Can you work these out from the model? Positions are in its coordinate system, mm. Face numbers are marked on the shaded views. A direction names the side the tool comes from. Round coordinates to 2 decimals unless told otherwise and drop trailing zeros. Loops run counter-clockwise (first coordinate to the right, second up) from the corner with the lowest first, then second, coordinate; pieces in that order, holes last.
```python
from build123d import *

# Parameters (mm, degrees)
F0_W      = 20
F0_H      = 20
F1_DEPTH  = 70
F0_W_2    = 5
F0_R      = 2.5
F2_DEPTH  = 5
F3_W      = 18
F3_H      = 18
F4_DEPTH  = 20
F5_W      = 20
F5_H      = 20
F6_DEPTH  = 2
F7_SIZE   = 2
F8_SIZE   = 1
F9_W      = 18
F9_H      = 18
F10_DEPTH = 20
F11_SIZE  = 1


with BuildPart() as f1:
    # F0 (on Top) → F1 (new body)
    with BuildSketch(Plane.XY):
        with Locations((15, 10)):
            Rectangle(F0_W, F0_H)
    extrude(amount=F1_DEPTH)

    # F0 (on Top) → F2 (join)
    with BuildSketch(Plane.XY):
        with Locations((2.5, 10)):
            Rectangle(F0_W_2, F0_H)
        with BuildLine():
            ThreePointArc((0, 20), (-10, 10), (0, 0))
            Line((0, 0), (0, 20))
        make_face()
        with Locations((-4, 10)):
            Circle(F0_R, mode=Mode.SUBTRACT)
        with Locations((15, 10)):
            Rectangle(F0_W, F0_H)
        with Locations((27.5, 10)):
            Rectangle(F0_W_2, F0_H)
        with BuildLine():
            Line((30, 20), (30, 0))
            ThreePointArc((30, 0), (40, 10), (30, 20))
        make_face()
        with Locations((34, 10)):
            Circle(F0_R, mode=Mode.SUBTRACT)
    extrude(amount=-F2_DEPTH)

    # F3 (on face) → F4 (join)
    with BuildSketch(Plane.XY.offset(70)):
        with Locations((15, 10)):
            Rectangle(F3_W, F3_H)
    extrude(amount=F4_DEPTH)

    # F5 (on face) → F6 (join)
    with BuildSketch(Plane.XZ):
        with Locations((15, 58)):
            Rectangle(F5_W, F5_H)
    extrude(amount=F6_DEPTH)

    # F7
    f7_edges = [f1.edges().sort_by_distance(p)[0] for p in [
        (31.5, 10, 0),
        (-6.5, 10, 0),
    ]]
    chamfer(f7_edges, length=F7_SIZE)

    # F8
    f8_edges = [f1.edges().sort_by_distance(p)[0] for p in [
        (24, 19, 80),
        (6, 19, 80),
        (15, 19, 90),
        (6, 10, 90),
        (24, 10, 90),
        (15, 1, 90),
        (24, 1, 80),
        (6, 1, 80),
    ]]
    chamfer(f8_edges, length=F8_SIZE)

    # F9 (on face) → F10 (join)
    with BuildSketch(Plane.XZ.offset(2)):
        with Locations((15, 58)):
            Rectangle(F9_W, F9_H)
    extrude(amount=F10_DEPTH)

    # F11
    f11_edges = [f1.edges().sort_by_distance(p)[0] for p in [
        (24, -12, 67),
        (15, -22, 67),
        (6, -12, 67),
        (24, -22, 58),
        (24, -12, 49),
        (6, -12, 49),
        (6, -22, 58),
        (15, -22, 49),
    ]]
    chamfer(f11_edges, length=F11_SIZE)


solid = f1.part
```
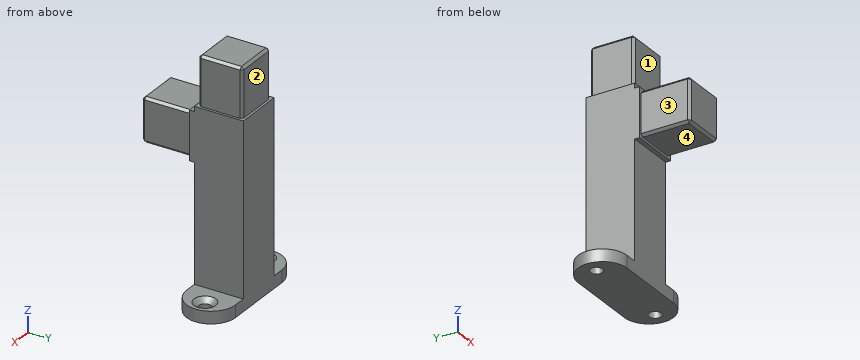
(1) Which directions (+Z, -Z, +X, -X, +Y, -Y) give clear straight access to the entire face, cutting with the end or side of a thin tool? Please do the marked faces 1, 2, 3 and 4.
(2) Suppose I cut it at C-C (y = -6). Write out the boundary of the cut face in (x, z).
(3) For pin 1 (4 mm diameter, centred on y = 9.5, z = 11, fed in from +X); pin 2 (5 mm diameter, centred on y = 10, z = 82.5, fed in from -X); pin 3 (24 mm diameter, centred on y = 5, z = 30.5, fed in from -X), each with a flat end and sliding along its axis, tell me the tip position at first contact or that it passes through.
(4) Suppose I cut it at D-D (x = 14). Write out the boundary of the cut face in (y, z), then the cut area to 3 significant figures.
(5) Suppose I cut it at B-B (x = -4). Write out the boundary of the cut face in (y, z).
(6) Suppose I cut it at A-A (y = 10). Write out the boundary of the cut face in (x, z).
(7) If I drill on line 1 (Z direction, x = 30.5, y = 7); line 2 (Y direction, x = 23, z = 5.5); line 3 (Y direction, x = 18.5, z = 81.5), over which ranges is the centre line in solid material (lowest first)?
Check result:
1. face 1: +Z, +X, -X, -Y
1. face 2: +Z, +X, -X, +Y
1. face 3: +Z, -Z, -X, -Y
1. face 4: -Z, +X, -X, -Y
2. outline: (6, 50) - (7, 49) - (23, 49) - (24, 50) - (24, 66) - (23, 67) - (7, 67) - (6, 66) - close
3. pin 1: stops at x = 25
3. pin 2: stops at x = 6
3. pin 3: stops at x = 5
4. outline: (-22, 50) - (-21, 49) - (-2, 49) - (-2, 48) - (0, 48) - (0, -5) - (20, -5) - (20, 70) - (19, 70) - (19, 89) - (18, 90) - (2, 90) - (1, 89) - (1, 70) - (0, 70) - (0, 68) - (-2, 68) - (-2, 67) - (-21, 67) - (-22, 66) - close
4. area: 2,260 mm2
5. outline: (0.83, -5) - (7.5, -5) - (7.5, -2) - (5.5, 0) - (0.83, 0) - close; (12.5, -5) - (19.17, -5) - (19.17, 0) - (14.5, 0) - (12.5, -2) - close
6. outline: (-10, -5) - (-6.5, -5) - (-6.5, -2) - (-8.5, 0) - (-10, 0) - close; (-1.5, -5) - (31.5, -5) - (31.5, -2) - (29.5, 0) - (25, 0) - (25, 70) - (24, 70) - (24, 89) - (23, 90) - (7, 90) - (6, 89) - (6, 70) - (5, 70) - (5, 0) - (0.5, 0) - (-1.5, -2) - close; (36.5, -5) - (40, -5) - (40, 0) - (38.5, 0) - (36.5, -2) - close
7. line 1: z = -5 to 0
7. line 2: y = 0 to 20
7. line 3: y = 1 to 19
